```python
from build123d import *

# Parameters (mm, degrees)
F0_W     = 57.15
F0_H     = 31.75
F1_DEPTH = 38.1
F2_W     = 25.4
F2_H     = 31.75
F3_DEPTH = 12.7
F4_DEPTH = 12.7
F6_DEPTH = 12.7
F8_DEPTH = 12.7


with BuildPart() as f1:
    # F0 (on Front) → F1 (new body)
    with BuildSketch(Plane.XZ):
        with Locations((28.575, 15.875)):
            Rectangle(F0_W, F0_H)
    extrude(amount=F1_DEPTH)

    # F2 (on face) → F3 (cut)
    with BuildSketch(Plane.XZ.offset(38.1)):
        with Locations((44.45, 15.875)):
            Rectangle(F2_W, F2_H)
    extrude(amount=-F3_DEPTH, mode=Mode.SUBTRACT)

    # F2 (on face) → F4 (cut)
    with BuildSketch(Plane.XZ.offset(38.1)):
        Polygon((18.840961, 31.75), (31.75, 0), (31.75, 31.75), align=None)
    extrude(amount=-F4_DEPTH, mode=Mode.SUBTRACT)

    # F5 (on face) → F6 (cut)
    with BuildSketch(Plane.XZ.offset(25.4)):
        Polygon((44.240961, 31.75), (57.15, 0), (57.15, 31.75), align=None)
    extrude(amount=-F6_DEPTH, mode=Mode.SUBTRACT)

    # F7 (on face) → F8 (cut)
    with BuildSketch(Plane(origin=(0, 0, 0), x_dir=(-1, 0, 0), z_dir=(0, 1, 0))):
        Polygon((-57.15, 0), (-31.75, 0), (-18.975182, 31.75), (-57.15, 31.75), align=None)
    extrude(amount=-F8_DEPTH, mode=Mode.SUBTRACT)


solid = f1.part
```
Design review of the part built by this model. Coordinates are the model's own, in mm. A direction names the side the tool comes from. Coordinates: 2 decimals unless noted, no trailing zeros. Order: outer loops, then holes, each group sorted by start corner. A loop starts at its lowest first (then second) coordinate and runs counter-clockwise, first axis right, second up. Notation, with made-up numbers: (-28, -12) -> (-15, -12) arc R28 cw to (-15, 21) -> close; hole circle Ø3 at (-13, -30). An arc over 180 degrees is marked (long way). One line per item, written item: value. Start each with the question number.
Q1. Insertion check: pin 1 Ø5 at (x, z) = (44.5, 10.5) entering from +Y; pin 2 Ø2 at (y, z) = (-30, 28.5) entering from +X; pin 3 Ø9.5 at (x, z) = (46, 11.5) entering from -Y. Each pin has a flat end and moves straight along its axis. Give the tip position at first contact, or say it passes through.
Q2. Tool access review of faces 1 (the flat face through (25.205, -31.839, 16.097)), 2 (the flat face through (17, -19, 31.75)), 3 (the flat face through (38, -12.7, 16)): name each direction out of +Z, -Z, +X, -X, +Y, -Y from which nothing blocks a thin tool from reaching the whole face with its end or side.
Q3. Take a section at C-C, the plane x = 43. State the section outline as (y, z) points.
Q4. Take a section at A-A, the plane z = 11.5. State the section outline as (x, y) points, then the cut area to 3 significant figures.
Q5. Take a section at B-B, the plane y = -22. State the section outline as (x, z) points.
Q6. Take a section at D-D, the plane z = 25. State the section outline as (x, y) points.
Q7. For probe 1 along Y at (x, z) = (34, 16); probe 2 along X at (y, z) = (-31.5, 23); probe 3 along X at (y, z) = (-35, 13), list the stretches that pass through material, from the lowest coordinate up.
Values follow:
1. pin 1: stops at y = -12.7
1. pin 2: stops at x = 20.57
1. pin 3: stops at y = -25.4
2. face 1: +Z, +X, -Y
2. face 2: +Z, +X, -X, +Y, -Y
2. face 3: +Z, +X, +Y
3. outline: (-25.4, 0) -> (-12.7, 0) -> (-12.7, 31.75) -> (-25.4, 31.75) -> close
4. outline: (0, -38.1) -> (27.07, -38.1) -> (27.07, -25.4) -> (52.47, -25.4) -> (52.47, -12.7) -> (27.12, -12.7) -> (27.12, 0) -> (0, 0) -> close
4. area: 1,350 mm2
5. outline: (0, 0) -> (57.15, 0) -> (44.24, 31.75) -> (0, 31.75) -> close
6. outline: (0, -38.1) -> (21.59, -38.1) -> (21.59, -25.4) -> (46.99, -25.4) -> (46.99, -12.7) -> (21.69, -12.7) -> (21.69, 0) -> (0, 0) -> close
7. probe 1: y = -25.4 to -12.7
7. probe 2: x = 0 to 22.4
7. probe 3: x = 0 to 26.46
